Can you work these out from the drawing? Everything is in mm from the part's minimum corner. Round coordinates to 2 decimals unless told otherwise and drop trailing zeros. Order: outer loops, then holes, each group sorted by start corner. A loop starts at its lowest first (then second) coordinate and runs counter-clockwise, first axis right, second up. Notation, with made-up numbers: (68, 1.25) - (83, 1.25) arc R18 ccw to (83, 18.25) - close; hole circle Ø6 at (-33.75, 47). An arc over 180 degrees is marked (long way). Answer as a JSON object with one key per item and string values.
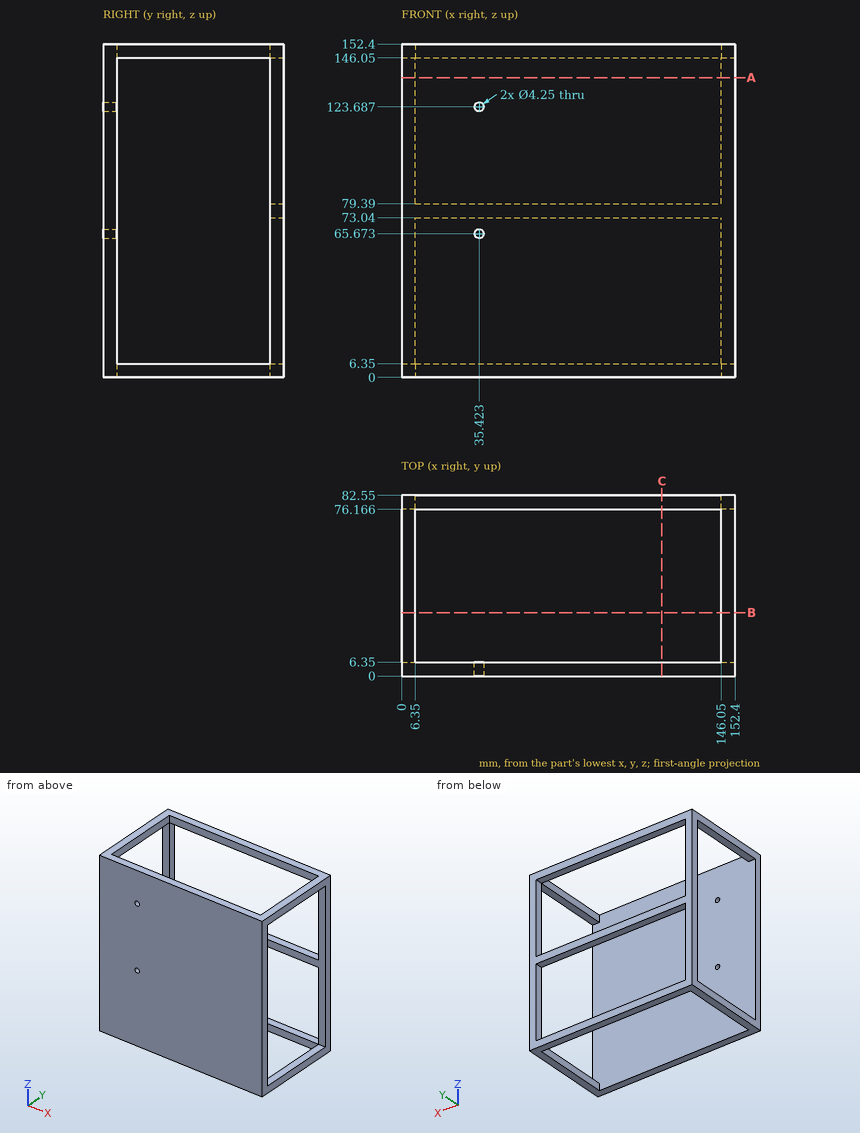
1. Imagine slicing it at A-A (z = 137). List the corners of the cut face in (x, y) for me, plus the area to 3 significant figures.
Responses:
{"outline": "(0, 0) - (152.4, 0) - (152.4, 6.35) - (0, 6.35) - close; (0, 76.17) - (6.35, 76.17) - (6.35, 82.55) - (0, 82.55) - close; (146.05, 76.17) - (152.4, 76.17) - (152.4, 82.55) - (146.05, 82.55) - close", "area": "1,050 mm2"}
2. Imagine slicing it at C-C (x = 119). List the corners of the cut face in (y, z) for me.
Responses:
{"outline": "(0, 0) - (6.35, 0) - (6.35, 152.4) - (0, 152.4) - close; (76.17, 0) - (82.55, 0) - (82.55, 6.35) - (76.17, 6.35) - close; (76.17, 73.04) - (82.55, 73.04) - (82.55, 79.39) - (76.17, 79.39) - close; (76.17, 146.05) - (82.55, 146.05) - (82.55, 152.4) - (76.17, 152.4) - close"}
3. If I drill on L1, parallel to Z at x = 119.5, y = 78; L2, parallel to X at y = 76.5, z = 52; L3, parallel to Y at x = 19, z = 145.5, over which ranges is the centre line in solid material (lowest first)? Write a range as [from, to].
Responses:
{"L1": "[0, 6.35], [73.04, 79.39], [146.05, 152.4]", "L2": "[0, 6.35], [146.05, 152.4]", "L3": "[0, 6.35]"}
4. For P1, Ø5, axis at x = 80.5, z = 148.5, coming from the -Y side; P2, Ø5, axis at x = 72, z = 131, coming from the +Y side, each with a flat end and sliding along its axis, tell me the tip position at first contact or that it passes through.
Responses:
{"P1": "y = 0", "P2": "y = 6.35"}
5. Imagine slicing it at B-B (y = 29). List the corners of the cut face in (x, z) for me, plus the area to 3 significant figures.
Responses:
{"outline": "(0, 0) - (6.35, 0) - (6.35, 6.35) - (0, 6.35) - close; (0, 146.05) - (6.35, 146.05) - (6.35, 152.4) - (0, 152.4) - close; (146.05, 0) - (152.4, 0) - (152.4, 6.35) - (146.05, 6.35) - close; (146.05, 146.05) - (152.4, 146.05) - (152.4, 152.4) - (146.05, 152.4) - close", "area": "161 mm2"}
